The listing builds one solid part. Answer for the finished solid, in the listing's coordinates (mm). A direction names the side the tool comes from. Coordinates: 2 decimals unless noted, no trailing zeros. Loops run counter-clockwise (first coordinate to the right, second up) from the corner with the lowest first, then second, coordinate; pieces in that order, holes last. Notation, with made-up numbers: M 56.25,43 L 105.25,43 A16 ccw 105.25,68 Z; hole C 83,-13 d4. An arc over 180 degrees is marked long. Answer as a JSON object with one key per item and string values. Group by question number.
1. Determine the mould class of faces 5 (the face through (289, 0, -14)), 6 (the face through (176, 0, -35)), 7 (the face through (0, 15, -2)), 8 (the face through (289, 0, 0)) for opening direction Z: released by +Z, released by -Z, zero draft, split by the parting line, or undercut.
2. Straight lines are drawn through the part: L1, parallel to Y at x = 297, z = 19; L2, parallel to Y at x = 154, z = 1.5; L3, parallel to X at y = -1, z = -4. For each, find the intervals that lie inside material, in ascending order.
3. Given pin 1 (5 mm diameter, centred on x = 0, z = 0, fed in from -Y); pin 2 (25 mm diameter, centred on y = 2.5, z = -13.5, fed in from -X); pin 3 (4 mm diameter, centred on y = 11, z = -19, fed in from +X) (3 decimals), each flat-ended and moving along its own axis, determine where each tip first touches the part or whether it passes through.
4. For faces 1 (the face through (179, 0, 35)), 2 (the face through (-18.5, 0.2, -0.1)), 3 (the face through (54.613, 20, 0)), 4 (the face through (172, 0, -30)), determine the directions among +Z, -Z, +X, -X, +Y, -Y from which every point of the face is accessible in a straight line to the end or side of a thin tool.
5. A cutting plane is placed at B-B on x = 79. Give the vertices of the cut face in (y, z).
6. A cutting plane is placed at A-A on x = 28.5. Give the vertices of the cut face in (y, z).
from build123d import *

# Parameters (mm, degrees)
SKETCH2_W                   = 20
SKETCH2_H                   = 30
SKETCH2_W_2                 = 14
SKETCH2_H_2                 = 24
BOSS_EXTRUDE1_DEPTH         = 302
SKETCH9_W                   = 70
SKETCH9_H                   = 60
BOSS_EXTRUDE2_DEPTH         = 3
BOSS_EXTRUDE3_DEPTH         = 9
BOSS_EXTRUDE3_DEPTH_BACK    = 9
SKETCH10_R                  = 21
SKETCH10_R_2                = 18.5
CUT_EXTRUDE1_DEPTH          = 19
CUT_EXTRUDE1_DEPTH_BACK     = 19
SKETCH14_W                  = 70
SKETCH14_H                  = 60
BOSS_EXTRUDE5_DEPTH         = 10
BOSS_EXTRUDE6_REACH         = 315.409
BOSS_EXTRUDE6_END_RADIUS    = 57.5
SKETCH15_W                  = 70
SKETCH15_H                  = 60
SKETCH15_W_2                = 60
SKETCH15_H_2                = 50
SKETCH16_W                  = 247.387457627
SKETCH16_H                  = 20
BOSS_EXTRUDE7_DEPTH         = 10
FILLET1_R                   = 5
M4_TAPPED_HOLE1_D           = 3.3
M4_TAPPED_HOLE1_DEPTH       = 8.008579979
M4_TAPPED_HOLE1_CSINK_D     = 4.05
M4_TAPPED_HOLE1_CSINK_ANGLE = 90
M4_TAPPED_HOLE1_TIP         = 0.991420021
SKETCH19_R                  = 1.525
CUT_EXTRUDE3_DEPTH          = 10


with BuildPart() as part:
    # Sketch2 → Boss-Extrude1 (new body)
    with BuildSketch(Plane(origin=(0, 0, 0), x_dir=(0, 0, -1), z_dir=(1, 0, 0))):
        Rectangle(SKETCH2_W, SKETCH2_H)
        Rectangle(SKETCH2_W_2, SKETCH2_H_2, mode=Mode.SUBTRACT)
    extrude(amount=BOSS_EXTRUDE1_DEPTH)

    # Sketch9 → Boss-Extrude2 (add)
    with BuildSketch(Plane(origin=(302, 0, 0), x_dir=(0, 0, -1), z_dir=(1, 0, 0))):
        Rectangle(SKETCH9_W, SKETCH9_H)
    extrude(amount=-BOSS_EXTRUDE2_DEPTH)

    # Sketch10 → Boss-Extrude3 (add, two sides: drawn at the far end of the back side and taken through both)
    # profile 1 of 3: a face of its own
    with BuildSketch(Plane.XY.offset(-BOSS_EXTRUDE3_DEPTH_BACK)):
        Circle(SKETCH10_R)
        Circle(SKETCH10_R_2, mode=Mode.SUBTRACT)
    # profile 2 of 3: a face of its own
    with BuildSketch(Plane.XY.offset(-BOSS_EXTRUDE3_DEPTH_BACK)):
        with BuildLine():
            ThreePointArc((10.828203914, 15), (0, 18.5), (-10.828203914, 15))
            Line((-10.828203914, 15), (10.828203914, 15))
        make_face()
    # profile 3 of 3: a face of its own
    with BuildSketch(Plane.XY.offset(-BOSS_EXTRUDE3_DEPTH_BACK)):
        with BuildLine():
            ThreePointArc((-10.828203914, -15), (0, -18.5), (10.828203914, -15))
            Line((10.828203914, -15), (-10.828203914, -15))
        make_face()
    extrude(amount=BOSS_EXTRUDE3_DEPTH + BOSS_EXTRUDE3_DEPTH_BACK)

    # Sketch10<3> → Cut-Extrude1 (cut, two sides: drawn at the far end of the back side and taken through both)
    with BuildSketch(Plane.XY.offset(-CUT_EXTRUDE1_DEPTH_BACK)):
        with BuildLine():
            Line((-10.828203914, -15), (10.828203914, -15))
            ThreePointArc((10.828203914, -15), (16.470758519, -8.42402005), (18.5, 0))
            ThreePointArc((18.5, 0), (16.470758519, 8.42402005), (10.828203914, 15))
            Line((10.828203914, 15), (-10.828203914, 15))
            ThreePointArc((-10.828203914, 15), (-18.5, 0), (-10.828203914, -15))
        make_face()
    extrude(amount=CUT_EXTRUDE1_DEPTH + CUT_EXTRUDE1_DEPTH_BACK, mode=Mode.SUBTRACT)

    # Sketch14 → Boss-Extrude5 (add)
    with BuildSketch(Plane.ZY.offset(-299)):
        Rectangle(SKETCH14_W, SKETCH14_H)
    extrude(amount=BOSS_EXTRUDE5_DEPTH)

    # Boss-Extrude6: up to this cylinder (the profile starts outside it)
    boss_extrude6_end = Plane(origin=(0, 0, 0), z_dir=(0, 0, -1)) * Cylinder(BOSS_EXTRUDE6_END_RADIUS, 746.818, mode=Mode.PRIVATE)
    # Sketch15 → Boss-Extrude6 (add, up to the surface)
    with BuildSketch(Plane.ZY.offset(-289), mode=Mode.PRIVATE) as boss_extrude6_sk1:
        Rectangle(SKETCH15_W, SKETCH15_H)
        Rectangle(SKETCH15_W_2, SKETCH15_H_2, mode=Mode.SUBTRACT)
    boss_extrude6_tool1 = extrude(boss_extrude6_sk1.sketch, amount=BOSS_EXTRUDE6_REACH, mode=Mode.PRIVATE) - boss_extrude6_end
    add(boss_extrude6_tool1.solids().sort_by_distance((289, -29.078046, 0))[0])

    # Sketch16 → Boss-Extrude7 (add)
    with BuildSketch(Plane(origin=(0, 15, 0), x_dir=(1, 0, 0), z_dir=(0, 1, 0))):
        with Locations((178.306271186, 0)):
            Rectangle(SKETCH16_W, SKETCH16_H)
    extrude(amount=BOSS_EXTRUDE7_DEPTH)

    # Fillet1
    fillet1_edges = [part.edges().sort_by_distance(p)[0] for p in [
        (302, -30, 0),
        (302, 0, -35),
        (175.526771088, -30, 35),
        (302, 30, 0),
        (175.526771088, 30, 35),
        (175.526771088, 30, -35),
        (175.526771088, -30, -35),
    ]]
    fillet(fillet1_edges, radius=FILLET1_R)

    # M4 Tapped Hole1
    with Locations(Plane(origin=(302, 0, 0), x_dir=(0, 0, -1), z_dir=(1, 0, 0))):
        with Locations((-19, 11), (19, 11), (-19, -11), (19, -11)):
            CounterSinkHole(M4_TAPPED_HOLE1_D / 2, M4_TAPPED_HOLE1_CSINK_D / 2, depth=M4_TAPPED_HOLE1_DEPTH, counter_sink_angle=M4_TAPPED_HOLE1_CSINK_ANGLE)
            with Locations((0, 0, -(M4_TAPPED_HOLE1_DEPTH + M4_TAPPED_HOLE1_TIP / 2))):  # 118° drill point
                Cone(0, M4_TAPPED_HOLE1_D / 2, M4_TAPPED_HOLE1_TIP, mode=Mode.SUBTRACT)

    # Sketch19 → Cut-Extrude3 (cut)
    with BuildSketch(Plane.XZ.offset(-15)):
        with Locations(Location((0, 0, 0), (0, 0, 270))):
            Circle(SKETCH19_R)
    extrude(amount=-CUT_EXTRUDE3_DEPTH, mode=Mode.SUBTRACT)


solid = part.part
From the geometry:
{
 "1": {"face 5": "undercut", "face 6": "released by -Z", "face 7": "zero draft", "face 8": "undercut"},
 "2": {"L1": "y = -30 to -12.65, -9.35 to 9.35, 12.65 to 30", "L2": "y = -30 to -25, -15 to -12, 12 to 30", "L3": "x = -20.98 to -18.47, 18.47 to 20.98, 289 to 302"},
 "3": {"pin 1": "stops at y = -21", "pin 2": "stops at x = -21", "pin 3": "stops at x = 301.975"},
 "4": {"face 1": "+Z, +X, -X, +Y, -Y", "face 2": "+Z, -Z", "face 3": "none", "face 4": "-X"},
 "5": {"outline": "M -30,-30 A5 ccw -25,-35 L 25,-35 A5 ccw 30,-30 L 30,30 A5 ccw 25,35 L -25,35 A5 ccw -30,30 Z; hole M -25,-30 L 25,-30 L 25,-10 L -15,-10 L -15,10 L 25,10 L 25,30 L -25,30 Z; hole M -12,-7 L 12,-7 L 12,7 L -12,7 Z"},
 "6": {"outline": "M -15,-10 L 15,-10 L 15,10 L -15,10 Z; hole M -12,-7 L 12,-7 L 12,7 L -12,7 Z"}
}
